Part print with two shaded views. Sizes in mm from the minimum x, y, z corner. A direction names the side the tool comes from. Give positions to 0.01 mm unless a question says otherwise; leave off trailing zeros. Write each loop counter-clockwise with the first axis right and the second up, starting at its lowest first coordinate (ties: lowest second). Pieces come first, ordered by that corner, then holes.
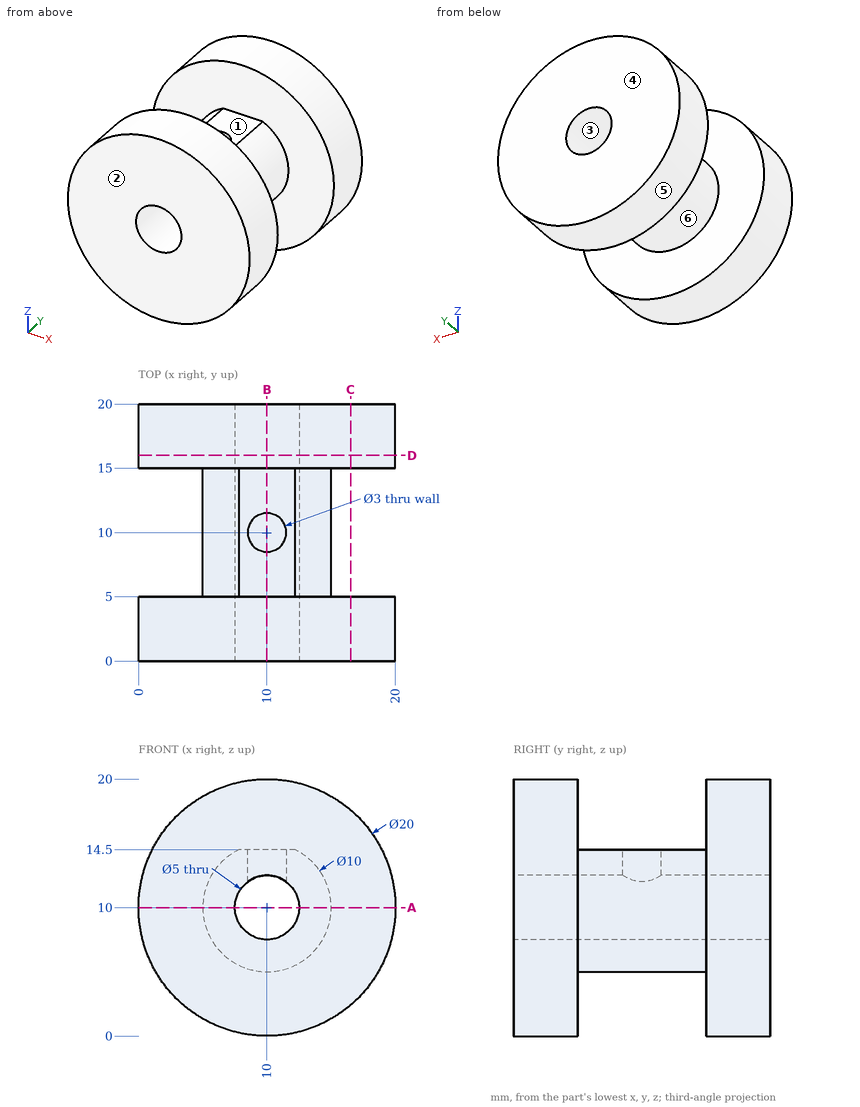
1) Saw through at A-A (z = 10). Write the cut outline in (x, y), and give its area (3 significant figures).
Check result:
outline: (0, 0) - (7.5, 0) - (7.5, 20) - (0, 20) - (0, 15) - (5, 15) - (5, 5) - (0, 5) - close; (12.5, 0) - (20, 0) - (20, 5) - (15, 5) - (15, 15) - (20, 15) - (20, 20) - (12.5, 20) - close
area: 200 mm2
2) Drill centre lines: L1, parallel to Y at x = 10, z = 13.7; L2, parallel to X at y = 6.25, z = 10; L3, parallel to Y at x = 16.75, z = 9.25. Where is each one in solid material? Low to high.
Check result:
L1: y = 0 to 8.5, 11.5 to 20
L2: x = 5 to 7.5, 12.5 to 15
L3: y = 0 to 5, 15 to 20
3) Saw through at D-D (y = 16). Write the cut outline in (x, z).
Check result:
outline: circle Ø20 at (10, 10); hole circle Ø5 at (10, 10)
4) Flat gauge pins, fed straight in: P1, Ø3.5, axis at x = 11, y = 10.5, coming from the +Z side; P2, Ø12, axis at y = 13, z = 17, coming from the -X side; P3, Ø4, axis at y = 2.5, z = 6.5, coming from the +X side. Where does each tip first touch, or does it go through?
Check result:
P1: stops at z = 14.5
P2: stops at x = 0.09
P3: stops at x = 19.89
5) Saw through at C-C (x = 16.5). Write the cut outline in (y, z), and give its area (3 significant figures).
Check result:
outline: (0, 2.4) - (5, 2.4) - (5, 17.6) - (0, 17.6) - close; (15, 2.4) - (20, 2.4) - (20, 17.6) - (15, 17.6) - close
area: 152 mm2
6) Saw through at B-B (x = 10). Write the cut outline in (y, z), and give its area (3 significant figures).
Check result:
outline: (0, 0) - (5, 0) - (5, 5) - (15, 5) - (15, 0) - (20, 0) - (20, 7.5) - (0, 7.5) - close; (0, 12.5) - (8.5, 12.5) - (8.5, 14.5) - (5, 14.5) - (5, 20) - (0, 20) - close; (11.5, 12.5) - (20, 12.5) - (20, 20) - (15, 20) - (15, 14.5) - (11.5, 14.5) - close
area: 189 mm2
7) Mould opens along Y. For the marked faces 1, 2, 3 and 4 say: +Y half, -Y half, draft (parallel to the pull), parting line (faces both ways), or undercut.
Check result:
face 1: undercut
face 2: -Y half
face 3: draft
face 4: +Y half
8) 3-axis set-ups, long thin cutter, end or side, ignore diameter. For the marked faces 5 and 6: which of +Z, -Z, +X, -X, +Y, -Y reach the whole face in a straight line?
Check result:
face 5: +Y, -Y
face 6: none
